Print and shaded views of the part. All mm, measured from the part's lowest x, y and z. A direction names the side the tool comes from. Give positions to 0.01 mm unless a question says otherwise; leave off trailing zeros. Order: outer loops, then holes, each group sorted by start corner. A loop starts at its lowest first (then second) coordinate and runs counter-clockwise, first axis right, second up. Notation, with made-up numbers: (36, 72.25) - (41, 72.25) arc R32 cw to (41, 111.25) - close; hole circle Ø6 at (-38, 39). An arc over 180 degrees is marked (long way). Answer in a Markdown table with one row per item.
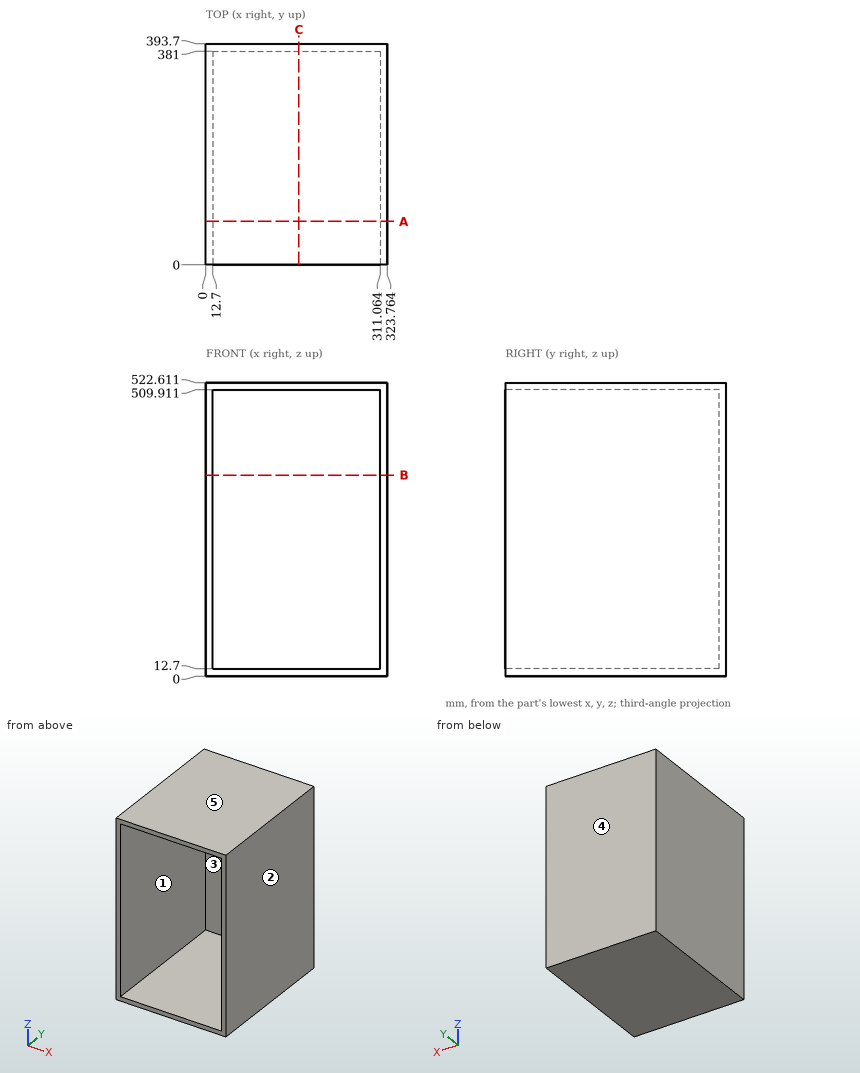
1. Two-plate mould, pull along Z, no slides. Class the marked faces 3, 4 and 5: +Z half, -Z half, draft (parallel to the pull), parting line (faces both ways), or undercut.
Check result:
| item | result |
|---|---|
| face 3 | undercut |
| face 4 | draft |
| face 5 | +Z half |
2. Probe line 1 (Z direction, x = 241, y = 203); line 2 (X direction, y = 352.5, z = 81); line 3 (Y direction, x = 31.5, z = 154.5). List the from-to ranges inside material, lowest first.
Check result:
| item | result |
|---|---|
| line 1 | z = 0 to 12.7, 509.91 to 522.61 |
| line 2 | x = 0 to 12.7, 311.06 to 323.76 |
| line 3 | y = 381 to 393.7 |
3. Cut at C-C on x = 166. Write the cut outline in (y, z).
Check result:
| item | result |
|---|---|
| outline | (0, 0) - (393.7, 0) - (393.7, 522.61) - (0, 522.61) - (0, 509.91) - (381, 509.91) - (381, 12.7) - (0, 12.7) - close |
4. Cut at B-B on z = 358. Write the cut outline in (x, y), and give its area (3 significant figures).
Check result:
| item | result |
|---|---|
| outline | (0, 0) - (12.7, 0) - (12.7, 381) - (311.06, 381) - (311.06, 0) - (323.76, 0) - (323.76, 393.7) - (0, 393.7) - close |
| area | 13,800 mm² |
5. Cut at A-A on y = 77.5. Write the cut outline in (x, z).
Check result:
| item | result |
|---|---|
| outline | (0, 0) - (323.76, 0) - (323.76, 522.61) - (0, 522.61) - close; hole (12.7, 12.7) - (311.06, 12.7) - (311.06, 509.91) - (12.7, 509.91) - close |
6. Drop a flat-ended pin along its axis: P1, Ø3, axis at x = 207.5, z = 383, coming from the -Y side. Give the stop position or say it passes through.
Check result:
| item | result |
|---|---|
| P1 | stops at y = 381 |
7. Which spindle directions (+Z, -Z, +X, -X, +Y, -Y) get a long thin tool onto all of the face, cutting with end or side? Do the marked faces 1 and 2. Say none if no direction does.
Check result:
| item | result |
|---|---|
| face 1 | -Y |
| face 2 | +Z, -Z, +X, +Y, -Y |
